Verification items for the finished model (mm, model axes). A direction names the side the tool comes from. Coordinates: 2 decimals unless noted, no trailing zeros. Write each loop counter-clockwise with the first axis right and the second up, starting at its lowest first coordinate (ties: lowest second). Pieces come first, ordered by that corner, then holes. Notation, with made-up numbers: M 38.5,-32 L 56.5,-32 A18 ccw 56.5,-2 Z; hole C 54.5,2 d1. An arc over 180 degrees is marked long. One line per item, written item: value.
Autodesk Inventor part; units mm, degrees
ref_plane "YZ Plane" through (0, 0, 0) normal (1, 0, 0) x (0, 1, 0)
ref_plane "XZ Plane" through (0, 0, 0) normal (0, 1, 0) x (-1, 0, 0)
ref_plane "XY Plane" through (0, 0, 0) normal (0, 0, 1) x (1, 0, 0)
sketch "Sketch1" plane through (0, 0, 0) normal (0, 1, 0) x (-1, 0, 0)
  line L0 (0, 0) -> (-127, 0)
  line L1 (-127, 0) -> (-127, -165.1)
  line L2 (-127, -165.1) -> (0, -165.1)
  line L3 (0, -165.1) -> (0, 0)
  dimension "d0" = 127
  dimension "d1" = 165.1
extrude "Extrusion1" add sketch "Sketch1" along normal blind 25.4
sketch "Sketch2" plane through (0, 25.4, 0) normal (0, 1, 0) x (1, 0, 0)
  circle A0 centre (82.55, 44.45) radius 25.4
  line L0 (0, 0) -> (127, 0)
  line L1 (127, 0) -> (127, 165.1)
  line L2 (127, 165.1) -> (0, 165.1)
  line L3 (0, 165.1) -> (0, 0)
  dimension "d4" = 50.8
  dimension "d5" = 44.45
  dimension "d6" = 44.45
extrude "Extrusion2" cut sketch "Sketch2" against normal blind 3.175 contours A0
sketch "Sketch3" plane through (82.55, 22.225, -44.45) normal (0, 1, 0) x (1, 0, 0)
  circle A0 centre (0, 0) radius 19.812
  point P0 (-82.55, -44.45)
  dimension "d9" = 39.624
extrude "Extrusion3" cut sketch "Sketch3" against normal blind 3.937
equation "\"d5\" = d6"
properties part number "AK plaque"
Item 1: Access from +Z, -Z, +X, -X, +Y, -Y to the whole of each face (thin tool, end or side, straight path). Record for faces 1 (the face through (62.393, 23.835, -28.994)), 2 (the face through (64, 0, -81)).
The answers:
face 1: +Y
face 2: +Z, -Z, +X, -X, -Y
Item 2: Draft check along Z on faces 3 (the face through (69.3, 22.225, -29.5)), 4 (the face through (63, 13, 0)), 5 (the face through (64, 13, -165.1)), 6 (the face through (64, 25.4, -81)). Enter one of: released by +Z, released by -Z, zero draft, split by the parting line, or undercut.
The answers:
face 3: undercut
face 4: released by +Z
face 5: released by -Z
face 6: zero draft
Item 3: Cross-section at A-A, the plane x = 82.55. Enter the section's corners in (y, z) (3 decimals), and give its area (3 significant figures).
The answers:
outline: M 0,-165.1 L 25.4,-165.1 L 25.4,-69.85 L 22.225,-69.85 L 22.225,-64.262 L 18.288,-64.262 L 18.288,-24.638 L 22.225,-24.638 L 22.225,-19.05 L 25.4,-19.05 L 25.4,0 L 0,0 Z
area: 3,880 mm²
Item 4: Scan lines: line 1 (X direction, y = 20.15, z = -44.45); line 2 (Z direction, x = 82.55, y = 20.95); line 3 (X direction, y = 23.6, z = -44.45). Record each from-to range of solid material in increasing order.
The answers:
line 1: x = 0 to 62.74, 102.36 to 127
line 2: z = -165.1 to -64.26, -24.64 to 0
line 3: x = 0 to 57.15, 107.95 to 127
Item 5: Cross-section at B-B, the plane z = -44.45. Enter the section's corners in (x, y) (3 decimals).
The answers:
outline: M 0,0 L 127,0 L 127,25.4 L 107.95,25.4 L 107.95,22.225 L 102.362,22.225 L 102.362,18.288 L 62.738,18.288 L 62.738,22.225 L 57.15,22.225 L 57.15,25.4 L 0,25.4 Z
